```python
from build123d import *

# Parameters (mm, degrees)
SKETCH_R        = 7
PAD_DEPTH       = 5
SKETCH001_R     = 8.5
SKETCH001_W     = 6.2
SKETCH001_H     = 20
POCKET_DEPTH    = 2.5
FILLET_R        = 4
FILLET001_R     = 4
POCKET001_DEPTH = 2.4
SKETCH003_R     = 1.7
POCKET002_DEPTH = 2.4
FILLET002_R     = 4
FILLET003_R     = 4
FILLET004_R     = 4
FILLET005_R     = 4
FILLET006_R     = 1


with BuildPart() as part:
    # Sketch → Pad (new body)
    with BuildSketch(Plane.XY):
        Polygon((-12.5, -12.5), (12.5, -12.5), (12.5, 12.5), (9, 25.5), (-9, 25.5), (-12.5, 12.5), align=None)
        Circle(SKETCH_R, mode=Mode.SUBTRACT)
    extrude(amount=PAD_DEPTH)

    # Sketch001 → Pocket (cut)
    with BuildSketch(Plane(origin=(0, 0, 0), x_dir=(1, 0, 0), z_dir=(0, 0, -1))):
        Circle(SKETCH001_R)
        with Locations((0, -20)):
            Rectangle(SKETCH001_W, SKETCH001_H)
    extrude(amount=-POCKET_DEPTH, mode=Mode.SUBTRACT)

    # Fillet
    fillet_edges = [part.edges().sort_by_distance(p)[0] for p in [
        (-12.5, -12.5, 2.5),
    ]]
    fillet(fillet_edges, radius=FILLET_R)

    # Fillet001
    fillet001_edges = [part.edges().sort_by_distance(p)[0] for p in [
        (12.5, -12.5, 2.5),
    ]]
    fillet(fillet001_edges, radius=FILLET001_R)

    # Sketch002 → Pocket001 (cut)
    with BuildSketch(Plane.XY.offset(5)):
        Polygon((-9.616581, 11.3), (-11.233162, 8.5), (-9.616581, 5.7), (-6.383419, 5.7), (-4.766838, 8.5), (-6.383419, 11.3), align=None)
        Polygon((6.383419, 11.3), (4.766838, 8.5), (6.383419, 5.7), (9.616581, 5.7), (11.233162, 8.5), (9.616581, 11.3), align=None)
        Polygon((-9.616581, -5.7), (-11.233162, -8.5), (-9.616581, -11.3), (-6.383419, -11.3), (-4.766838, -8.5), (-6.383419, -5.7), align=None)
        Polygon((6.383419, -5.7), (4.766838, -8.5), (6.383419, -11.3), (9.616581, -11.3), (11.233162, -8.5), (9.616581, -5.7), align=None)
        Polygon((-7.616581, 22.8), (-9.233162, 20), (-7.616581, 17.2), (-4.383419, 17.2), (-2.766838, 20), (-4.383419, 22.8), align=None)
        Polygon((4.383419, 22.8), (2.766838, 20), (4.383419, 17.2), (7.616581, 17.2), (9.233162, 20), (7.616581, 22.8), align=None)
    extrude(amount=-POCKET001_DEPTH, mode=Mode.SUBTRACT)

    # Sketch003 → Pocket002 (cut)
    with BuildSketch(Plane(origin=(0, 0, 0), x_dir=(1, 0, 0), z_dir=(0, 0, -1))):
        with Locations((-8, 8.5)):
            Circle(SKETCH003_R)
        with Locations((8, 8.5)):
            Circle(SKETCH003_R)
        with Locations((-8, -8.5)):
            Circle(SKETCH003_R)
        with Locations((8, -8.5)):
            Circle(SKETCH003_R)
        with Locations((-6, -20)):
            Circle(SKETCH003_R)
        with Locations((6, -20)):
            Circle(SKETCH003_R)
    extrude(amount=-POCKET002_DEPTH, mode=Mode.SUBTRACT)

    # Fillet002
    fillet002_edges = [part.edges().sort_by_distance(p)[0] for p in [
        (12.5, 12.5, 2.5),
    ]]
    fillet(fillet002_edges, radius=FILLET002_R)

    # Fillet003
    fillet003_edges = [part.edges().sort_by_distance(p)[0] for p in [
        (-12.5, 12.5, 2.5),
    ]]
    fillet(fillet003_edges, radius=FILLET003_R)

    # Fillet004
    fillet004_edges = [part.edges().sort_by_distance(p)[0] for p in [
        (-9, 25.5, 2.5),
    ]]
    fillet(fillet004_edges, radius=FILLET004_R)

    # Fillet005
    fillet005_edges = [part.edges().sort_by_distance(p)[0] for p in [
        (9, 25.5, 2.5),
    ]]
    fillet(fillet005_edges, radius=FILLET005_R)

    # Fillet006
    fillet006_edges = [part.edges().sort_by_distance(p)[0] for p in [
        (11.079707, 17.775373, 5),
    ]]
    fillet(fillet006_edges, radius=FILLET006_R)


solid = part.part
```
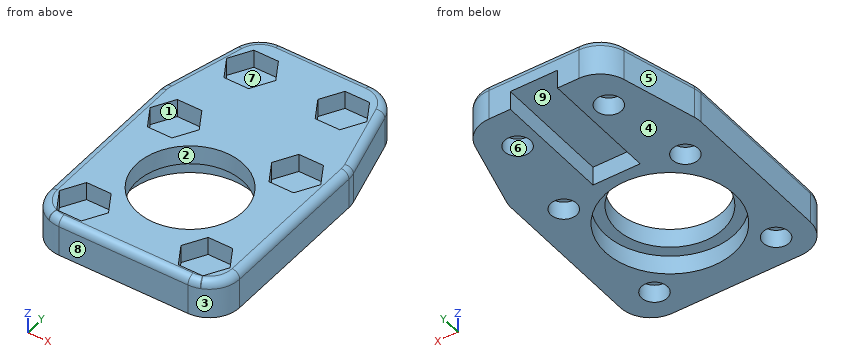
CAD build for the part. Positions are in the model's coordinates, mm. Face numbers are marked on the shaded views. A direction names the side the tool comes from. Round coordinates to 2 decimals unless told otherwise and drop trailing zeros. Order: outer loops, then holes, each group sorted by start corner. A loop starts at its lowest first (then second) coordinate and runs counter-clockwise, first axis right, second up. Notation, with made-up numbers: (56, 12) - (97, 12) arc R14 cw to (97, 23) - close; hole circle Ø1 at (70.5, 65.5). An arc over 180 degrees is marked (long way). Answer in a Markdown table with one row per item. Add a question column.
(1) Drop flat-ended pins along their axis: pin 1 Ø0.8 at (x, z) = (-1.5, 1) entering from +Y; pin 2 Ø1.2 at (x, z) = (8.5, 4.5) entering from +Y; pin 3 Ø1.5 at (y, z) = (19, 4) entering from +X. Give the stop position or say it passes through.
(2) Mould opens along X. For the marked faces 1, 2, 3 and 4 say: +X half, -X half, draft (parallel to the pull), parting line (faces both ways), or undercut.
(3) 3-axis set-ups, long thin cutter, end or side, ignore diameter. For the marked faces 5, 6, 7, 8 and 9: which of +Z, -Z, +X, -X, +Y, -Y reach the whole face in a straight line?
(4) Probe L1, parallel to X at y = 0, z = 3.85; L2, parallel to X at y = 20.5, z = 3.8; L3, parallel to Y at x = 3.75, z = 2.65. List the from-to ranges inside material, lowest first. Write a range as [from, to].
(5) Band-saw the part on A-A on y = 0. List the corners of the cut face in (x, z).
(6) Band-saw the part on C-C on y = 9. List the corners of the cut face in (x, z).
(7) Band-saw the part on B-B on x = 0. List the corners of the cut face in (y, z).
Data:
| question | item | result |
|---|---|---|
| 1 | pin 1 | stops at y = 10 |
| 1 | pin 2 | stops at y = 24.92 |
| 1 | pin 3 | stops at x = 10.95 |
| 2 | face 1 | undercut |
| 2 | face 2 | undercut |
| 2 | face 3 | +X half |
| 2 | face 4 | draft |
| 3 | face 5 | +Z, -Z, -X, +Y |
| 3 | face 6 | -Z |
| 3 | face 7 | +Z |
| 3 | face 8 | +Z, -Z, +X, -X, -Y |
| 3 | face 9 | -Z, +Y |
| 4 | L1 | x = [-12.5, -7], [7, 12.5] |
| 4 | L2 | x = [-10.35, -8.94], [-3.06, 3.06], [8.94, 10.35] |
| 4 | L3 | y = [-12.5, -5.91], [5.91, 18.3], [21.7, 25.5] |
| 5 | outline | (-12.5, 0) - (-8.5, 0) - (-8.5, 2.5) - (-7, 2.5) - (-7, 5) - (-11.5, 5) arc R1 ccw to (-12.5, 4) - close; (7, 2.5) - (8.5, 2.5) - (8.5, 0) - (12.5, 0) - (12.5, 4) arc R1 ccw to (11.5, 5) - (7, 5) - close |
| 6 | outline | (-12.5, 0) - (-9.62, 0) - (-9.62, 2.4) - (-6.38, 2.4) - (-6.38, 0) - (6.38, 0) - (6.38, 2.4) - (9.62, 2.4) - (9.62, 0) - (12.5, 0) - (12.5, 4) arc R1 ccw to (11.5, 5) - (10.94, 5) - (10.94, 2.6) - (5.06, 2.6) - (5.06, 5) - (-5.06, 5) - (-5.06, 2.6) - (-10.94, 2.6) - (-10.94, 5) - (-11.5, 5) arc R1 ccw to (-12.5, 4) - close |
| 7 | outline | (-12.5, 0) - (-8.5, 0) - (-8.5, 2.5) - (-7, 2.5) - (-7, 5) - (-11.5, 5) arc R1 ccw to (-12.5, 4) - close; (7, 2.5) - (8.5, 2.5) - (8.5, 0) - (10, 0) - (10, 2.5) - (25.5, 2.5) - (25.5, 4) arc R1 ccw to (24.5, 5) - (7, 5) - close |
